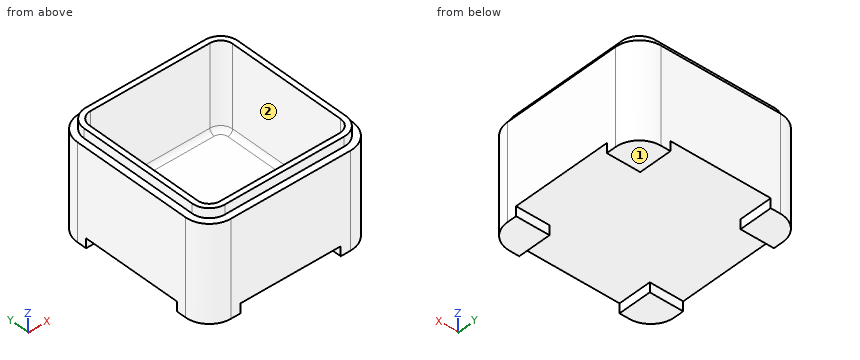
```python
from build123d import *

# Parameters (mm, degrees)
F0_W         = 35
F0_H         = 35
F1_DEPTH     = 11
F2_W         = 21
F2_H         = 7
F2_W_2       = 7
F2_H_2       = 21
F3_DEPTH     = 2
F4_W         = 35
F4_H         = 35
F4_W_2       = 32.2
F4_H_2       = 32.2
F5_DEPTH     = 2
F6_W         = 30
F6_H         = 30
F7_DEPTH     = 18
F8_R         = 1
F9_T1_DEPTH  = 18
F9_T4_ANGLE  = 90
F9_T6_ANGLE  = 90
F9_T8_ANGLE  = 90
F9_T10_ANGLE = 90
F10_R        = 3.6
F11_R        = 5


# Not quite as in the source:
# - a fillet or chamfer that OpenCascade refuses, or shapes differently, is made with other operations: its cross-section is extruded or revolved along the edge and cut away or added


with BuildPart() as f1:
    # F0 (on Top) → F1 (new body, symmetric)
    with BuildSketch(Plane.XY):
        Rectangle(F0_W, F0_H)
    extrude(amount=F1_DEPTH, both=True)

    # F2 (on face) → F3 (cut)
    with BuildSketch(Plane(origin=(0, 0, -11), x_dir=(1, 0, 0), z_dir=(0, 0, -1))):
        with Locations((0, -14)):
            Rectangle(F2_W, F2_H)
        with Locations((-14, 0)):
            Rectangle(F2_W_2, F2_H_2)
        Rectangle(F2_W, F2_H_2)
        with Locations((14, 0)):
            Rectangle(F2_W_2, F2_H_2)
        with Locations((0, 14)):
            Rectangle(F2_W, F2_H)
    extrude(amount=-F3_DEPTH, mode=Mode.SUBTRACT)

    # F4 (on face) → F5 (cut)
    with BuildSketch(Plane.XY.offset(11)):
        Rectangle(F4_W, F4_H)
        Rectangle(F4_W_2, F4_H_2, mode=Mode.SUBTRACT)
    extrude(amount=-F5_DEPTH, mode=Mode.SUBTRACT)

    # F6 (on face) → F7 (cut)
    with BuildSketch(Plane.XY.offset(11)):
        Rectangle(F6_W, F6_H)
    extrude(amount=-F7_DEPTH, mode=Mode.SUBTRACT)

    # F8
    f8_edges = [f1.edges().sort_by_distance(p)[0] for p in [
        (0, 15, -7),
        (-15, 0, -7),
        (0, -15, -7),
        (15, 0, -7),
    ]]
    fillet(f8_edges, radius=F8_R)

    # F9: fillet of radius 2.5 on 4 edges, made by hand

    # F9_s2 → F9_t1 (join)
    with BuildSketch(Plane.XY.offset(-7)):
        with BuildLine():
            ThreePointArc((-12.5, 15), (-14.267766953, 14.267766953), (-15, 12.5))
            Line((-15, 12.5), (-15, 15))
            Line((-15, 15), (-12.5, 15))
        make_face()
        with BuildLine():
            ThreePointArc((15, -12.5), (14.267766953, -14.267766953), (12.5, -15))
            Line((12.5, -15), (15, -15))
            Line((15, -15), (15, -12.5))
        make_face()
        with BuildLine():
            ThreePointArc((15, 12.5), (14.267766953, 14.267766953), (12.5, 15))
            Line((12.5, 15), (15, 15))
            Line((15, 15), (15, 12.5))
        make_face()
        with BuildLine():
            ThreePointArc((-12.5, -15), (-14.267766953, -14.267766953), (-15, -12.5))
            Line((-15, -12.5), (-15, -15))
            Line((-15, -15), (-12.5, -15))
        make_face()
    extrude(amount=F9_T1_DEPTH)

    # F9_s3 → F9_t4 (revolve)
    with BuildSketch(Plane.YZ.offset(-12.5)):
        with BuildLine():
            ThreePointArc((-14, -7), (-14.7071067812, -6.7071067812), (-15, -6))
            Line((-15, -6), (-15, -7))
            Line((-15, -7), (-14, -7))
        make_face()
    revolve(axis=Axis((-12.5, -12.5, -7), (0, 0, -1)), revolution_arc=F9_T4_ANGLE)

    # F9_s5 → F9_t6 (revolve)
    with BuildSketch(Plane.YZ.offset(12.5)):
        with BuildLine():
            ThreePointArc((14, -7), (14.7071067812, -6.7071067812), (15, -6))
            Line((15, -6), (15, -7))
            Line((15, -7), (14, -7))
        make_face()
    revolve(axis=Axis((12.5, 12.5, -7), (0, 0, -1)), revolution_arc=F9_T6_ANGLE)

    # F9_s7 → F9_t8 (revolve)
    with BuildSketch(Plane.XZ.offset(12.5)):
        with BuildLine():
            ThreePointArc((14, -7), (14.7071067812, -6.7071067812), (15, -6))
            Line((15, -6), (15, -7))
            Line((15, -7), (14, -7))
        make_face()
    revolve(axis=Axis((12.5, -12.5, -7), (0, 0, -1)), revolution_arc=F9_T8_ANGLE)

    # F9_s9 → F9_t10 (revolve)
    with BuildSketch(Plane.XZ.offset(-12.5)):
        with BuildLine():
            ThreePointArc((-14, -7), (-14.7071067812, -6.7071067812), (-15, -6))
            Line((-15, -6), (-15, -7))
            Line((-15, -7), (-14, -7))
        make_face()
    revolve(axis=Axis((-12.5, 12.5, -7), (0, 0, -1)), revolution_arc=F9_T10_ANGLE)

    # F10
    f10_edges = [f1.edges().sort_by_distance(p)[0] for p in [
        (-16.1, -16.1, 10),
        (16.1, -16.1, 10),
        (16.1, 16.1, 10),
        (-16.1, 16.1, 10),
    ]]
    fillet(f10_edges, radius=F10_R)

    # F11
    f11_edges = [f1.edges().sort_by_distance(p)[0] for p in [
        (-17.5, -17.5, -1),
        (17.5, -17.5, -1),
        (17.5, 17.5, -1),
        (-17.5, 17.5, -1),
    ]]
    fillet(f11_edges, radius=F11_R)


solid = f1.part
```
Could you check a few things on this model? Use its own coordinates, in mm. Face numbers are marked on the shaded views. A direction names the side the tool comes from. Round coordinates to 2 decimals unless told otherwise and drop trailing zeros. Write each loop counter-clockwise with the first axis right and the second up, starting at its lowest first coordinate (ties: lowest second). Pieces come first, ordered by that corner, then holes.
(1) Which directions (+Z, -Z, +X, -X, +Y, -Y) give clear straight access to the entire face, cutting with the end or side of a thin tool? Please do the marked faces 1 and 2.
Findings below:
face 1: -Z, +X, -X, +Y, -Y
face 2: +Z
(2) Suppose I cut it at D-D on x = 11.5. Write out the boundary of the cut face in (y, z).
Findings below:
outline: (-17.5, -11) - (-10.5, -11) - (-10.5, -9) - (10.5, -9) - (10.5, -11) - (17.5, -11) - (17.5, 9) - (16.1, 9) - (16.1, 11) - (15, 11) - (15, -6) arc R1 cw to (14, -7) - (-14, -7) arc R1 cw to (-15, -6) - (-15, 11) - (-16.1, 11) - (-16.1, 9) - (-17.5, 9) - close
(3) Suppose I cut it at A-A on x = 2. Write out the boundary of the cut face in (y, z).
Findings below:
outline: (-17.5, -9) - (17.5, -9) - (17.5, 9) - (16.1, 9) - (16.1, 11) - (15, 11) - (15, -6) arc R1 cw to (14, -7) - (-14, -7) arc R1 cw to (-15, -6) - (-15, 11) - (-16.1, 11) - (-16.1, 9) - (-17.5, 9) - close
(4) For pin 1 (0.6 mm diameter, centred on y = 15, z = -10.5, fed in from +X); pin 2 (1.6 mm diameter, centred on x = -13.5, z = -9.5, fed in from +Y); pin 3 (5 mm diameter, centred on x = 1, y = 4, fed in from +Z), each with a flat end and sliding along its axis, tell me the tip position at first contact or that it passes through.
Findings below:
pin 1: stops at x = 16.99
pin 2: stops at y = 17.5
pin 3: stops at z = -7
(5) Suppose I cut it at B-B on z = -3.5. Write out the boundary of the cut face in (x, y).
Findings below:
outline: (-17.5, -12.5) arc R5 ccw to (-12.5, -17.5) - (12.5, -17.5) arc R5 ccw to (17.5, -12.5) - (17.5, 12.5) arc R5 ccw to (12.5, 17.5) - (-12.5, 17.5) arc R5 ccw to (-17.5, 12.5) - close; hole (-15, -12.5) arc R2.5 ccw to (-12.5, -15) - (12.5, -15) arc R2.5 ccw to (15, -12.5) - (15, 12.5) arc R2.5 ccw to (12.5, 15) - (-12.5, 15) arc R2.5 ccw to (-15, 12.5) - close
(6) If I drill on probe 1 along Y at (x, z) = (5, 8.25); probe 2 along X at (y, z) = (-0.5, 10.25), over which ranges is the centre line in solid material (lowest first)?
Findings below:
probe 1: y = -17.5 to -15, 15 to 17.5
probe 2: x = -16.1 to -15, 15 to 16.1
